Geometry: final body of the model. Coordinates: model frame, mm. Face numbers are marked on the shaded views. A direction names the side the tool comes from. Coordinates: 2 decimals unless noted, no trailing zeros. Loops run counter-clockwise (first coordinate to the right, second up) from the corner with the lowest first, then second, coordinate; pieces in that order, holes last. Notation, with made-up numbers: M 55,-14 L 80,-14 A29 ccw 80,13 Z; hole C -0.5,83.25 d10. An arc over 180 degrees is marked long. Write item = value, one per line. Start each with the question number.
```python
from build123d import *

# Parameters (mm, degrees)
SKETCH1_R           = 35
SKETCH1_R_2         = 24.188
BOSS_EXTRUDE1_DEPTH = 11
CHAMFER1_SIZE       = 4.5
CHAMFER1_SIZE2      = 2.598076211
CUT_EXTRUDE1_REACH  = 52.705
CUT_EXTRUDE2_REACH  = 52.705
CUT_EXTRUDE3_REACH  = 52.705
CUT_EXTRUDE4_REACH  = 52.616
CHAMFER2_SIZE       = 0.812
CHAMFER3_SIZE       = 0.812
FILLET1_R           = 1.833333333
FILLET2_R           = 1.833333333


with BuildPart() as part:
    # Sketch1 → Boss-Extrude1 (new body)
    with BuildSketch(Plane(origin=(0, 0, 0), x_dir=(0, -1, 0), z_dir=(-1, 0, 0))):
        with Locations(Location((0, 0, 0), (0, 0, 270))):
            Circle(SKETCH1_R)
        with Locations(Location((0, 0, 0), (0, 0, 270))):
            Circle(SKETCH1_R_2, mode=Mode.SUBTRACT)
    extrude(amount=-BOSS_EXTRUDE1_DEPTH)

    # Chamfer1
    chamfer1_edges = [part.edges().sort_by_distance(p)[0] for p in [
        (0, 0, 35),
    ]]
    chamfer1_side = [part.faces().sort_by_distance(p)[0] for p in [
        (0, 0, 34.010050506),
    ]]
    chamfer(chamfer1_edges, length=CHAMFER1_SIZE, length2=CHAMFER1_SIZE2, reference=chamfer1_side[0])

    # Cut-Extrude1: up to this cone (the profile starts inside it)
    cut_extrude1_end = Plane(origin=(11, 0, 0), z_dir=(1, 0, 0)).offset(-28.60918221) * Cone(1.732e-06, 227.533871731, 131.366741094, align=(Align.CENTER, Align.CENTER, Align.MIN), mode=Mode.PRIVATE)
    # Sketch2 → Cut-Extrude1 (cut, up to the surface)
    with BuildSketch(Plane(origin=(11, 0, 0), x_dir=(0, 0, -1), z_dir=(1, 0, 0)), mode=Mode.PRIVATE) as cut_extrude1_sk1:
        with BuildLine():
            Line((34.871191548, 3), (32.371191548, 3))
            Line((32.371191548, 3), (32.371191548, -3))
            Line((32.371191548, -3), (34.871191548, -3))
            ThreePointArc((34.871191548, -3), (35, 0), (34.871191548, 3))
        make_face()
    cut_extrude1_tool1 = extrude(cut_extrude1_sk1.sketch, amount=-CUT_EXTRUDE1_REACH, mode=Mode.PRIVATE) & cut_extrude1_end
    add(cut_extrude1_tool1.solids().sort_by_distance((11, 0, -33.664429))[0], mode=Mode.SUBTRACT)

    # Cut-Extrude2: up to this cone (the profile starts inside it)
    cut_extrude2_end = Plane(origin=(11, 0, 0), z_dir=(1, 0, 0)).offset(-28.60918221) * Cone(1.732e-06, 227.533871731, 131.366741094, align=(Align.CENTER, Align.CENTER, Align.MIN), mode=Mode.PRIVATE)
    # Sketch3 → Cut-Extrude2 (cut, up to the surface)
    with BuildSketch(Plane(origin=(11, 0, 0), x_dir=(0, 0, -1), z_dir=(1, 0, 0)), mode=Mode.PRIVATE) as cut_extrude2_sk1:
        with BuildLine():
            Line((3, -34.871191548), (3, -32.371191548))
            Line((3, -32.371191548), (-3, -32.371191548))
            Line((-3, -32.371191548), (-3, -34.871191548))
            ThreePointArc((-3, -34.871191548), (0, -35), (3, -34.871191548))
        make_face()
    cut_extrude2_tool1 = extrude(cut_extrude2_sk1.sketch, amount=-CUT_EXTRUDE2_REACH, mode=Mode.PRIVATE) & cut_extrude2_end
    add(cut_extrude2_tool1.solids().sort_by_distance((11, -33.664429, 0))[0], mode=Mode.SUBTRACT)

    # Cut-Extrude3: up to this cone (the profile starts inside it)
    cut_extrude3_end = Plane(origin=(11, 0, 0), z_dir=(1, 0, 0)).offset(-28.60918221) * Cone(1.732e-06, 227.533871731, 131.366741094, align=(Align.CENTER, Align.CENTER, Align.MIN), mode=Mode.PRIVATE)
    # Sketch4 → Cut-Extrude3 (cut, up to the surface)
    with BuildSketch(Plane(origin=(11, 0, 0), x_dir=(0, 0, -1), z_dir=(1, 0, 0)), mode=Mode.PRIVATE) as cut_extrude3_sk1:
        with BuildLine():
            Line((-34.871191548, -3), (-32.371191548, -3))
            Line((-32.371191548, -3), (-32.371191548, 3))
            Line((-32.371191548, 3), (-34.871191548, 3))
            ThreePointArc((-34.871191548, 3), (-35, 0), (-34.871191548, -3))
        make_face()
    cut_extrude3_tool1 = extrude(cut_extrude3_sk1.sketch, amount=-CUT_EXTRUDE3_REACH, mode=Mode.PRIVATE) & cut_extrude3_end
    add(cut_extrude3_tool1.solids().sort_by_distance((11, 0, 33.664429))[0], mode=Mode.SUBTRACT)

    # Cut-Extrude4: up to this cone (the profile starts inside it)
    cut_extrude4_end = Plane(origin=(11, 0, 0), z_dir=(1, 0, 0)).offset(-28.60918221) * Cone(1.732e-06, 227.379719209, 131.277741094, align=(Align.CENTER, Align.CENTER, Align.MIN), mode=Mode.PRIVATE)
    # Sketch5 → Cut-Extrude4 (cut, up to the surface)
    with BuildSketch(Plane(origin=(11, 0, 0), x_dir=(0, 0, -1), z_dir=(1, 0, 0)), mode=Mode.PRIVATE) as cut_extrude4_sk1:
        with BuildLine():
            Line((-3, 34.871191548), (-3, 32.371191548))
            Line((-3, 32.371191548), (3, 32.371191548))
            Line((3, 32.371191548), (3, 34.871191548))
            ThreePointArc((3, 34.871191548), (0, 35), (-3, 34.871191548))
        make_face()
    cut_extrude4_tool1 = extrude(cut_extrude4_sk1.sketch, amount=-CUT_EXTRUDE4_REACH, mode=Mode.PRIVATE) & cut_extrude4_end
    add(cut_extrude4_tool1.solids().sort_by_distance((11, 33.664429, 0))[0], mode=Mode.SUBTRACT)

    # Chamfer2
    chamfer2_edges = [part.edges().sort_by_distance(p)[0] for p in [
        (0, 0, 24.188),
    ]]
    chamfer(chamfer2_edges, length=CHAMFER2_SIZE)

    # Chamfer3
    chamfer3_edges = [part.edges().sort_by_distance(p)[0] for p in [
        (11, 0, 24.188),
    ]]
    chamfer(chamfer3_edges, length=CHAMFER3_SIZE)

    # Fillet1
    fillet1_edges = [part.edges().sort_by_distance(p)[0] for p in [
        (11, -24.748737342, 24.748737342),
        (11, 24.748737342, 24.748737342),
        (11, -24.748737342, -24.748737342),
    ]]
    fillet(fillet1_edges, radius=FILLET1_R)

    # Fillet2
    fillet2_edges = [part.edges().sort_by_distance(p)[0] for p in [
        (11, 24.748737342, -24.748737342),
    ]]
    fillet(fillet2_edges, radius=FILLET2_R)


solid = part.part
```
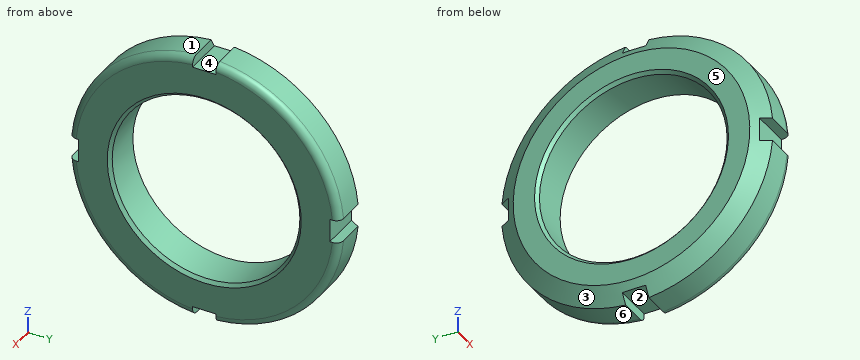
Item 1: First-contact query: pin 1 (3 mm diameter, centred on x = 8, y = 0, fed in from +Z); pin 2 (1.8 mm diameter, centred on x = 5, z = 0, fed in from +Y); pin 3 (2 mm diameter, centred on x = 3, z = 23, fed in from -Y). Flat tips, straight axial feed; report the tip coordinate or a pass-through.
Item 2: Section query A-A (z = 0). Return the cut outline in (x, y), plus the area to 3 significant figures.
Item 3: Pull-direction query (Y, two-part tool) for the marked faces 3, 4, 5 and 6; classes: released by +Y, released by -Y, zero draft, split by the parting line, or undercut.
Item 4: Line query: line 1 (Y direction, x = 3.5, z = 0); line 2 (Y direction, x = 3, z = 10); line 3 (Z direction, x = 0.5, y = 18.5). Output: solid intervals per line, ascending. Write a range as from..to.
Item 5: Section query B-B (x = 7.75). Return the cut outline in (y, z).
Item 6: Reachability of the marked faces 1 and 2 from +Z, -Z, +X, -X, +Y, -Y: full face, straight path, thin tool, end or side. Return the list, or none.
Verdict:
q1.pin_1 = 32.37
q1.pin_2 = 32.37
q1.pin_3 = -27.22
q2.outline = M 0,-30.5 L 1.08,-32.37 L 11,-32.37 L 11,-25 L 10.19,-24.19 L 0.81,-24.19 L 0,-25 Z; M 0,25 L 0.81,24.19 L 10.19,24.19 L 11,25 L 11,32.37 L 1.08,32.37 L 0,30.5 Z
q2.area = 177 mm2
q3.face_3 = split by the parting line
q3.face_4 = undercut
q3.face_5 = zero draft
q3.face_6 = released by +Y
q4.line_1 = -32.37..-24.19, 24.19..32.37
q4.line_2 = -33.54..-22.02, 22.02..33.54
q4.line_3 = -25.33..-16.06, 16.06..25.33
q5.outline = M -34.87,-3 A35 ccw -3,-34.87 L -3,-32.37 L 3,-32.37 L 3,-34.87 A35 ccw 34.87,-3 L 32.37,-3 L 32.37,3 L 34.87,3 A35 ccw 3,34.87 L 3,32.37 L -3,32.37 L -3,34.87 A35 ccw -34.87,3 L -32.37,3 L -32.37,-3 Z; hole C 0,0 d48.38
q6.face_1 = +Z, +X, -X, -Y
q6.face_2 = -Z, +X, -X
